```python
from build123d import *

# Parameters (mm, degrees)
F0_W      = 118
F0_H      = 95
F1_DEPTH  = 6
F2_W      = 118
F2_H      = 74
F3_DEPTH  = 6
F4_W      = 118
F4_H      = 6
F5_DEPTH  = 50
F7_DEPTH  = 118
F9_DEPTH  = 118.001
F11_R     = 21.25
F12_DEPTH = 5.3079525657


with BuildPart() as f1:
    # F0 (on Top) → F1 (new body)
    with BuildSketch(Plane.XY):
        Rectangle(F0_W, F0_H)
    extrude(amount=F1_DEPTH)

    # F2 (on face) → F3 (join)
    with BuildSketch(Plane(origin=(0, 47.5, 0), x_dir=(-1, 0, 0), z_dir=(0, 1, 0))):
        with Locations((0, 43)):
            Rectangle(F2_W, F2_H)
    extrude(amount=-F3_DEPTH)

    # F4 (on face) → F5 (join)
    with BuildSketch(Plane.XZ.offset(-41.5)):
        with Locations((0, 77)):
            Rectangle(F4_W, F4_H)
    extrude(amount=F5_DEPTH)

    # F6 (on face) → F7 (join)
    with BuildSketch(Plane(origin=(-59, 0, 0), x_dir=(0, -1, 0), z_dir=(-1, 0, 0))):
        Polygon((38.3378378378, 6), (44.3378378378, 6), (8.5, 74), (2.5, 74), align=None)
        Polygon((2.5, 74), (8.5, 74), (5.3378378378, 80), (-0.6621621622, 80), align=None)
        Polygon((41.5, 0), (47.5, 0), (44.3378378378, 6), (38.3378378378, 6), align=None)
    extrude(amount=-F7_DEPTH)

    # F8 (on face) → F9 (cut, through all)
    with BuildSketch(Plane.YZ.offset(59)):
        Polygon((-47.5, 6), (-47.5, 0), (-44.3378378378, 6), align=None)
        Polygon((-8.5, 80), (-8.5, 74), (-5.3378378378, 80), align=None)
    extrude(amount=-F9_DEPTH, mode=Mode.SUBTRACT)

    # F11 (on face) → F12 (cut, through all)
    with BuildSketch(Plane(origin=(0, -37.1745033586, 19.5919679863), x_dir=(1, 0, 0), z_dir=(0, -0.884658761, 0.4662390767))):
        with Locations((-29.2115788907, 25.8900932968)):
            Circle(F11_R)
        with Locations((29.2115788907, 25.8900932968)):
            Circle(F11_R)
    extrude(amount=-F12_DEPTH, mode=Mode.SUBTRACT)


solid = f1.part
```
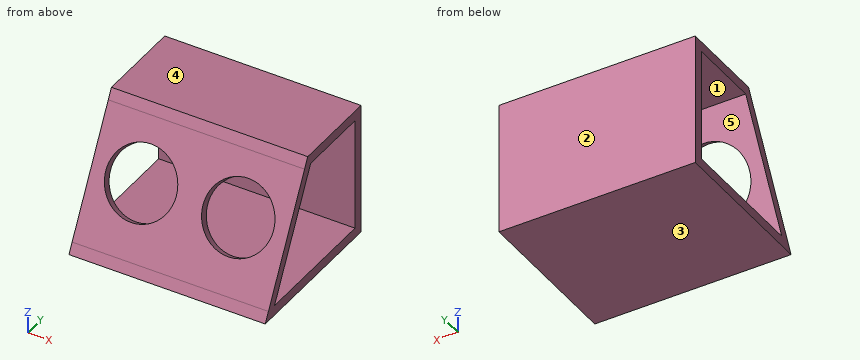
Geometry: final body of the model. Coordinates: model frame, mm. Face numbers are marked on the shaded views. A direction names the side the tool comes from. Coordinates: 2 decimals unless noted, no trailing zeros. Loops run counter-clockwise (first coordinate to the right, second up) from the corner with the lowest first, then second, coordinate; pieces in that order, holes last. Notation, with made-up numbers: (-5, -14.5) -> (46, -14.5) arc R32 ccw to (46, 16.5) -> close; hole circle Ø4 at (25.5, 23.5). An arc over 180 degrees is marked (long way). Use a Markdown table: item, result. Add a question column.
(1) Section query C-C, the plane z = 69. Return loops of the section in (x, y).
(2) Access query for the marked faces 1 and 2. Directions: +Z, -Z, +X, -X, +Y, -Y. A direction counts if a zero-diameter tool reaches every point of the face in a straight line with its end or side. Return the directions, or none.
(3) Mould query, pull axis Z, two halves, no side actions, for the marked faces 3, 4 and 5. Classes: pulls with the +Z half, pulls with the -Z half, needs draft (parallel to the pull), parting line crosses it, or undercut.
(4) Section query D-D, the plane x = -23. Return loops of the section in (y, z).
(5) Pin query (flat end, axial travel): pin 1 Ø8 at (y, z) = (-1, 64) entering from -X; pin 2 Ø1 at (x, y) = (-0.5, -26) entering from -Z. Return the tip coordinate at first contact, or that it passes through.
(6) Section query B-B, the plane x = -1. Return loops of the section in (y, z), plus the area to 3 significant figures.
(7) Line query: line 1 along Z through (x, y) = (-40.5, 4); line 2 along Y through (x, z) = (-33.5, 27); line 3 along Z through (x, y) = (-25, -14.5). Output: solid intervals per line, ascending.
(8) Section query A-A, the plane y = 0. Return loops of the section in (x, z), plus the area to 3 significant figures.
Answer:
| question | item | result |
|---|---|---|
| 1 | outline | (-59, -11.14) -> (59, -11.14) -> (59, -5.14) -> (-59, -5.14) -> close; (-59, 41.5) -> (59, 41.5) -> (59, 47.5) -> (-59, 47.5) -> close |
| 2 | face 1 | +X, -X |
| 2 | face 2 | +Z, -Z, +X, -X, +Y |
| 3 | face 3 | pulls with the -Z half |
| 3 | face 4 | pulls with the +Z half |
| 3 | face 5 | undercut |
| 4 | outline | (-47.5, 0) -> (47.5, 0) -> (47.5, 80) -> (-5.34, 80) -> (-15.63, 60.47) -> (-10.93, 58) -> (-2.5, 74) -> (41.5, 74) -> (41.5, 6) -> (-38.34, 6) -> (-29.88, 22.04) -> (-34.58, 24.52) -> close |
| 5 | pin 1 | passes through |
| 5 | pin 2 | stops at z = 0 |
| 6 | outline | (-47.5, 0) -> (47.5, 0) -> (47.5, 80) -> (-5.34, 80) -> close; hole (-38.34, 6) -> (41.5, 6) -> (41.5, 74) -> (-2.5, 74) -> close |
| 6 | area | 1,700 mm^2 |
| 7 | line 1 | z = 0 to 6, 74 to 80 |
| 7 | line 2 | y = 41.5 to 47.5 |
| 7 | line 3 | z = 0 to 6, 60.45 to 62.62 |
| 8 | outline | (-59, 0) -> (59, 0) -> (59, 6) -> (-59, 6) -> close; (-59, 74) -> (59, 74) -> (59, 80) -> (-59, 80) -> close |
| 8 | area | 1,420 mm^2 |
